Design review of the part built by this model. Coordinates are the model's own, in mm. A direction names the side the tool comes from. Give positions to 0.01 mm unless a question says otherwise; leave off trailing zeros. Loops run counter-clockwise (first coordinate to the right, second up) from the corner with the lowest first, then second, coordinate; pieces in that order, holes last. Notation, with made-up numbers: M -19,-3 L -14,-3 A13 cw -14,10 Z; hole C 21,46.5 d6. An arc over 180 degrees is marked long. Use a Markdown table: item, result. Add a question column.
(1) Draft analysis for pull direction X (two halves, no side actions). For faces 4 (the face through (-3.4, -16, 3.9)), 5 (the face through (6, 6, 9.6)), 6 (the face through (3.4, 5, 6)), state which applies: pulls with the +X half, pulls with the -X half, needs draft (parallel to the pull), parting line crosses it, or undercut.
(2) Add section C-C, the plane z = 1.5. State how many separate pieces and enclosed holes the cut face has, then the cut area to 3 significant figures.
(3) For probe 1 along Y at (x, z) = (-3.5, 5.75); probe 2 along X at (y, z) = (10.5, 5.75); probe 3 along X at (y, z) = (7, 2.75), list the stretches that pass through material, from the lowest coordinate up.
(4) Insertion check: pin 1 Ø2.5 at (x, z) = (-9, 5) entering from -Y; pin 2 Ø4 at (x, y) = (-13, -3) entering from -Z; pin 3 Ø3 at (x, z) = (-6, 8.5) entering from +Y. Each pin has a flat end and moves straight along its axis. Give the tip position at first contact, or say it passes through.
(5) Add section A-A, the plane x = -3.5. Give the boundary of the cut face in (y, z), then the cut area to 3 significant figures.
(6) Add section B-B, the plane y = 10.5. Give the boundary of the cut face in (x, z), then the cut area to 3 significant figures.
(7) For faces 1 (the face through (2, 23, 4)), 2 (the face through (-10.4, 6, 5)), 3 (the face through (-11, 6, 8)), list the 3-axis set-ups (+Z, -Z, +X, -X, +Y, -Y) from which the entire face can be reached by the end or side of a thin tool; tool diameter is ignored.
(8) Add section D-D, the plane z = 5. Give the boundary of the cut face in (x, y), then the cut area to 3 significant figures.
Autodesk Fusion 360 part; units mm, degrees
sketch "Skizze1" plane through (0, 0, 0) normal (0, 0, 1) x (1, 0, 0)
  circle A0 centre (-13, 14) radius 1.6
  circle A1 centre (-13, -3) radius 1.6
  line L0 (-10.4, 17) -> (-10.4, -6)
  line L1 (-11.4, 14) -> (-10.4, 14) construction
  line L2 (-19, 17) -> (14, 17)
  line L3 (-20.3748, -6) -> (15.4156, -6)
  line L4 (-16.4, 27.5706) -> (-16.4, -12)
  line L5 (-11.401, -2.9445) -> (3.799, -2.9445) construction
  line L6 (3.4, -14.6443) -> (3.4, 27)
  line L7 (9.4, 27) -> (9.4, -17)
  line L8 (-21, 23) -> (15, 23)
  line L9 (15, -12) -> (-27, -12)
  circle A2 centre (6, 10.5) radius 1.6
  line L10 (4.4, 10.5) -> (3.4, 10.5) construction
  line L11 (-13, -3) -> (-13, 3) construction
  line L12 (-13, 3) -> (-13, -17) construction
  line L13 (9.4, -17) -> (-16.4, -17) construction
  line L14 (-13, 3) -> (-13, 23) construction
  line L15 (-16.4, 22.0964) -> (9.4, 22.0964) construction
  line L16 (-3.5, 22.0964) -> (-3.5, 23) construction
  circle A3 centre (-3.5, 23) radius 2.05
  circle A4 centre (-3.5, 23) radius 4
  circle A5 centre (-3.5, -12) radius 2.05
  circle A6 centre (-3.5, -12) radius 4
  point P0 (-3.5, -17)
  point P1 (-3.5, 22.0964)
  dimension "d1" = 3.2
  dimension "d2" = 3.2
  dimension "d3" = 17
  dimension "d4" = 1
  dimension "d5" = 3
  dimension "d6" = 3
  dimension "d7" = 6
  dimension "d8" = 15.2
  dimension "d9" = 6
  dimension "d10" = 6
  dimension "d11" = 6
  dimension "d12" = 3.2
  dimension "d13" = 3.5
  dimension "d16" = 2.6
  dimension "d21" = 6
  dimension "d22" = 20
  dimension "d24" = 25.8
  dimension "d27" = 20
  dimension "d28" = 4.1
  dimension "d29" = 8
  dimension "d40" = 4.1
  dimension "d41" = 8
extrude "Extrusion1" add sketch "Skizze1" along normal blind 8 contours L0 L2 L3 L4 | L2 L4 L6 L8 A4 | L3 L4 L6 L9 A6 | L2 L6 L7 L8 | L2 L3 L6 L7 | L3 L6 L7 L9 | L8 A3 A4 | L9 A5 A6 | L8 A3 | L9 A5 picked at (-0.1725, 22.6994) picked at (-6.7682, -11.3064) picked at (-3.4489, 22.3186) picked at (-2.9991, -11.3315)
extrude "Extrusion2" add sketch "Skizze1" along normal blind 9.6 contours L2 L6 L7 L8 | L2 L3 L6 L7 | L3 L6 L7 L9
extrude "Extrusion3" add sketch "Skizze1" along normal blind 8 contours L8 A3 A4 | L9 A5 A6 picked at (-6.8275, 23.3006) picked at (-6.8351, -12.1987)
extrude "Extrusion7" cut sketch "Skizze1" along normal blind 8 contours L8 A3 | L9 A5 picked at (-3.4489, 22.3186) picked at (-2.9991, -11.3315)
fillet "Abrundung2" radius 6 4 edges at (-16.4, -12, 4) (-16.4, 23, 4) (9.4, 23, 4.8) (9.4, -12, 4.8)
sketch "Skizze2" plane through (0, 0, 0) normal (0, 0, -1) x (1, 0, 0)
  circle A0 centre (-13, -14) radius 1.6
  circle A1 centre (-13, 3) radius 1.6
  line L0 (3.4, 6) -> (3.4, -17)
  line L1 (3.4, -17) -> (-10.4, -17)
  line L2 (-10.4, -17) -> (-10.4, 6)
  line L3 (-10.4, 6) -> (3.4, 6)
  circle A2 centre (6, -10.5) radius 1.6
  arc A3 (9.4, 6) -> (3.4, 12) centre (3.4, 6) ccw
  line L4 (3.4, 12) -> (0.5, 12)
  arc A4 (0.5, 12) -> (-7.5, 12) centre (-3.5, 12) ccw
  line L5 (-7.5, 12) -> (-10.4, 12)
  arc A5 (-10.4, 12) -> (-16.4, 6) centre (-10.4, 6) ccw
  line L6 (-16.4, 6) -> (-16.4, -17)
  arc A6 (-16.4, -17) -> (-10.4, -23) centre (-10.4, -17) ccw
  line L7 (-10.4, -23) -> (-7.5, -23)
  arc A7 (-7.5, -23) -> (0.5, -23) centre (-3.5, -23) ccw
  line L8 (0.5, -23) -> (3.4, -23)
  arc A8 (3.4, -23) -> (9.4, -17) centre (3.4, -17) ccw
  line L9 (9.4, -17) -> (9.4, 6)
  circle A9 centre (-3.5, 12) radius 2.05
  circle A10 centre (-3.5, -23) radius 2.05
  circle A11 centre (-13, 3) radius 3
  circle A12 centre (-13, -14) radius 3
  circle A13 centre (6, -10.5) radius 3
  line L10 (-10, 3) -> (-10, 6)
  line L11 (-10, -14) -> (-10, -17)
  line L12 (-13, 6) -> (-10.4, 6)
  line L13 (-13, 0) -> (-10.4, 0)
  line L14 (6, -7.5) -> (3.4, -7.5)
  line L15 (-13, -11) -> (-10.4, -11)
  line L16 (-13, -17) -> (-10.4, -17)
  line L17 (6, -13.5) -> (3.4, -13.5)
  line L18 (-13, 6) -> (-16.4, 6)
  line L19 (-13, 0) -> (-16.4, 0)
  line L20 (6, -7.5) -> (9.4, -7.5)
  line L21 (6, -13.5) -> (9.4, -13.5)
  line L22 (-13, -17) -> (-16.4, -17)
  line L23 (-13, -11) -> (-16.4, -11)
  dimension "d46" = 1.4
  dimension "d47" = 1.4
  dimension "d48" = 1.4
extrude "Extrusion8" cut sketch "Skizze2" against normal blind 3 contours L0 A13 L14 | L0 A13 | L9 A13 L20 L21 | L2 A11 L12 | L0 A13 L17 | L2 A11 | L6 A11 L18 L19 | L2 A11 L13 | L2 A12 L15 | L6 A12 L22 L23 | L2 A12 | L2 A12 L16 picked at (3.7333, -10.5) picked at (-10.7333, 3) picked at (-10.7333, -14)
Established:
| question | item | result |
|---|---|---|
| 1 | face 4 | parting line crosses it |
| 1 | face 5 | needs draft |
| 1 | face 6 | undercut |
| 2 | separate pieces | 3 |
| 2 | enclosed holes | 2 |
| 2 | area | 471 mm^2 |
| 3 | probe 1 | -16 to -14.05, -9.95 to -6, 17 to 20.95, 25.05 to 27 |
| 3 | probe 2 | -16.4 to -10.4, 3.4 to 4.4, 7.6 to 9.4 |
| 3 | probe 3 | -16.4 to -10.4, 3.4 to 9.4 |
| 4 | pin 1 | y = -12 |
| 4 | pin 2 | z = 3 |
| 4 | pin 3 | y = 26.85 |
| 5 | outline | M -16,0 L -14.05,0 L -14.05,8 L -16,8 Z; M -9.95,0 L -6,0 L -6,8 L -9.95,8 Z; M 17,0 L 20.95,0 L 20.95,8 L 17,8 Z; M 25.05,0 L 27,0 L 27,8 L 25.05,8 Z |
| 5 | area | 94.4 mm^2 |
| 6 | outline | M -16.4,0 L -10.4,0 L -10.4,8 L -16.4,8 Z; M 3.4,3 L 4.4,3 L 4.4,9.6 L 3.4,9.6 Z; M 7.6,3 L 9.4,3 L 9.4,9.6 L 7.6,9.6 Z |
| 6 | area | 66.5 mm^2 |
| 7 | face 1 | +Z, -Z, +X, +Y |
| 7 | face 2 | +Z, -Z |
| 7 | face 3 | +Z, -X, +Y, -Y |
| 8 | outline | M -16.4,-6 A6 ccw -10.4,-12 L -7.5,-12 A4 ccw 0.5,-12 L 3.4,-12 A6 ccw 9.4,-6 L 9.4,17 A6 ccw 3.4,23 L 0.5,23 A4 ccw -7.5,23 L -10.4,23 A6 ccw -16.4,17 Z; hole C -13,-3 d3.2; hole C -13,14 d3.2; hole M -10.4,-6 L 3.4,-6 L 3.4,17 L -10.4,17 Z; hole C -3.5,-12 d4.1; hole C -3.5,23 d4.1; hole C 6,10.5 d3.2 |
| 8 | area | 554 mm^2 |
